Can you work these out from the model? Positions are in its coordinate system, mm. Face numbers are marked on the shaded views. A direction names the side the tool comes from. Round coordinates to 2 decimals unless told otherwise and drop trailing zeros. Order: outer loops, then holes, each group sorted by start corner. A loop starts at its lowest first (then second) coordinate and runs counter-clockwise, first axis right, second up. Notation, with made-up numbers: (-9.75, 50.25) - (10.25, 50.25) arc R19 ccw to (10.25, 64.25) - close; hole circle Ø5 at (9.25, 6.5). An arc over 180 degrees is marked (long way). Write item = value, one per line.
from build123d import *

# Parameters (mm, degrees)
LINEAR_AUSTRAGEN_D_NN1_DEPTH         = 15
VERRUNDUNG1_R                        = 1
SCHNITT_LINEAR_AUSTRAGEN2_DEPTH      = 73.284161474
SCHNITT_LINEAR_AUSTRAGEN2_DEPTH_BACK = 73.284161474
VERRUNDUNG2_R                        = 1


with BuildPart() as part:
    # Skizze1 → Linear-Austragen-Dünn1 (new body)
    with BuildSketch(Plane.XY):
        Polygon((-50, 0), (-42.5, 50), (42.5, 50), (50, 0), (48.022127294, -0.296680906), (40.777625158, 48), (-40.777625158, 48), (-48.022127294, -0.296680906), align=None)
    extrude(amount=LINEAR_AUSTRAGEN_D_NN1_DEPTH)

    # Verrundung1
    verrundung1_edges = [part.edges().sort_by_distance(p)[0] for p in [
        (0, 50, 15),
        (-49.011063647, -0.148340453, 15),
        (49.011063647, -0.148340453, 15),
    ]]
    fillet(verrundung1_edges, radius=VERRUNDUNG1_R)

    # Skizze2 → Schnitt-Linear austragen2 (cut, two sides: drawn at the far end of the back side and taken through both)
    with BuildSketch(Plane(origin=(0, 0, 0), x_dir=(0, 0, -1), z_dir=(1, 0, 0)).offset(-SCHNITT_LINEAR_AUSTRAGEN2_DEPTH_BACK)):
        Polygon((-15, 11.139702343), (-5, 7.5), (-5, 5), (-15, 8.639702343), align=None)
    extrude(amount=SCHNITT_LINEAR_AUSTRAGEN2_DEPTH + SCHNITT_LINEAR_AUSTRAGEN2_DEPTH_BACK, mode=Mode.SUBTRACT)

    # Verrundung2
    verrundung2_edges = [part.edges().sort_by_distance(p)[0] for p in [
        (-47.692857228, 8.639702343, 15),
        (47.692857228, 8.639702343, 15),
        (47.317857228, 11.139702343, 15),
        (-47.317857228, 11.139702343, 15),
    ]]
    fillet(verrundung2_edges, radius=VERRUNDUNG2_R)


solid = part.part
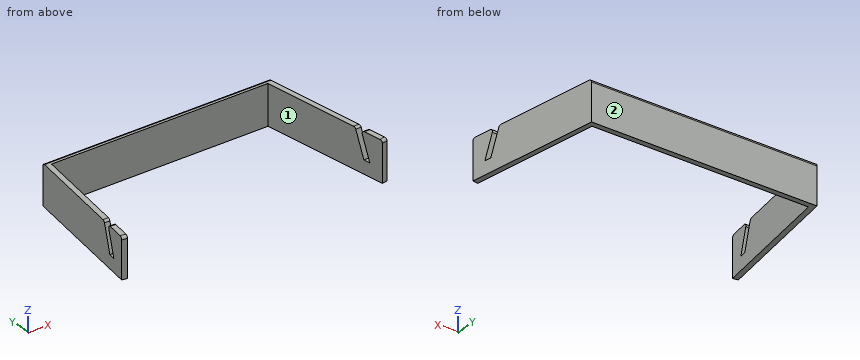
(1) If we section it at B-B (y = 22): Write out the boundary of the cut face in (x, z).
Computed:
outline = (-46.7, 0) - (-44.68, 0) - (-44.68, 15) - (-46.7, 15) - close; (44.68, 0) - (46.7, 0) - (46.7, 15) - (44.68, 15) - close
(2) Will these pins go through, and if not, where does the flat tip stop? P1, Ø3, axis at y = 16.5, z = 12.5, coming from the -X side; P2, Ø2, axis at y = 29.5, z = 12, coming from the +X side (3 decimals); P3, Ø12, axis at x = -24.5, y = 38.5, coming from the -Z side; P4, Ø4.5, axis at x = 17, z = 10.5, coming from the -Y side.
Computed:
P1 = -47.75
P2 = 45.725
P3 = through
P4 = 48
(3) If I drill on line 1 (X direction, y = 11, z = 13.5); line 2 (Y direction, x = -35.5, z = 4.25); line 3 (X direction, y = 37.5, z = 2.25) (3 decimals), over which ranges is the centre line in solid material (lowest first)? Write a range as from..to.
Computed:
line_1 = -48.35..-46.33, 46.33..48.35
line_2 = 48..50
line_3 = -44.375..-42.353, 42.353..44.375
(4) If we section it at A-A (z = 7): Write out the boundary of the cut face in (x, y).
Computed:
outline = (-50, 0) - (-48.02, -0.3) - (-47.12, 5.73) - (-49.14, 5.73) - close; (-48.77, 8.23) - (-46.74, 8.23) - (-40.78, 48) - (40.78, 48) - (46.74, 8.23) - (48.77, 8.23) - (42.5, 50) - (-42.5, 50) - close; (47.12, 5.73) - (48.02, -0.3) - (50, 0) - (49.14, 5.73) - close
(5) If we section it at C-C (x = 3.5): Write out the boundary of the cut face in (y, z).
Computed:
outline = (48, 0) - (50, 0) - (50, 14) arc R1 ccw to (49, 15) - (48, 15) - close
(6) On a 3-axis mill with a long thin cutter (end or side, diameter ignored), from which of +Z, -Z, +X, -X, +Y, -Y can I reach the whole of each face in a straight line? I mean the marked faces 1 and 2. Say none if no direction works.
Computed:
face_1 = +Z, -Z, -Y
face_2 = +Z, -Z, +X, -X, +Y
(7) If we section it at D-D (x = -44): Write out the boundary of the cut face in (y, z).
Computed:
outline = (26.52, 0) - (40, 0) - (40, 15) - (26.52, 15) - close
